Can you work these out from the model? Positions are in its coordinate system, mm. A direction names the side the tool comes from. Give positions to 0.01 mm unless a question says otherwise; leave off trailing zeros. Order: outer loops, then holes, each group sorted by start corner. A loop starts at its lowest first (then second) coordinate and runs counter-clockwise, first axis right, second up.
```python
from build123d import *

# Parameters (mm, degrees)
BOSS_EXTRUDE1_DEPTH     = 3
BOSS_EXTRUDE2_DEPTH     = 3.4
CUT_EXTRUDE1_DEPTH      = 1
CUT_EXTRUDE1_DEPTH_BACK = 8.35
CUT_EXTRUDE2_DEPTH      = 10.948718941
CUT_EXTRUDE2_DEPTH_BACK = 7
SKETCH6_R               = 1.5
SKETCH6_R_2             = 1
CUT_EXTRUDE4_DEPTH      = 1
CUT_EXTRUDE4_DEPTH_BACK = 8.35
FILLET1_R               = 10
FILLET2_R               = 3


with BuildPart() as part:
    # Sketch1 → Boss-Extrude1 (new body, symmetric)
    with BuildSketch(Plane.XY):
        Polygon((-14.712036777, 3.95), (8.397963223, 3.95), (28.677963223, 0), (-14.712036777, 0), align=None)
    extrude(amount=BOSS_EXTRUDE1_DEPTH, both=True)

    # Sketch2 → Boss-Extrude2 (add)
    with BuildSketch(Plane.XZ):
        with BuildLine():
            Line((-11.712036777, -3), (31.08325999, -3))
            Line((31.08325999, -3), (42.367258396, 7.779455791))
            ThreePointArc((42.367258396, 7.779455791), (42.464252889, 12.020987598), (38.222721082, 12.117982091))
            Line((38.222721082, 12.117982091), (28.677963223, 3))
            Line((28.677963223, 3), (-11.712036777, 3))
            ThreePointArc((-11.712036777, 3), (-14.712036777, 0), (-11.712036777, -3))
        make_face()
    extrude(amount=BOSS_EXTRUDE2_DEPTH)

    # Sketch3 → Cut-Extrude1 (cut, two sides)
    with BuildSketch(Plane(origin=(0, 3.95, 0), x_dir=(1, 0, 0), z_dir=(0, 1, 0))) as cut_extrude1_sk:
        with BuildLine():
            ThreePointArc((-14.712036777, 0), (-13.833357121, 2.121320344), (-11.712036777, 3))
            Line((-11.712036777, 3), (-14.712036777, 3))
            Line((-14.712036777, 3), (-14.712036777, 0))
        make_face()
        with BuildLine():
            ThreePointArc((-11.712036777, -3), (-13.833357121, -2.121320344), (-14.712036777, 0))
            Line((-14.712036777, 0), (-14.712036777, -3))
            Line((-14.712036777, -3), (-11.712036777, -3))
        make_face()
    extrude(amount=CUT_EXTRUDE1_DEPTH, mode=Mode.SUBTRACT)
    extrude(cut_extrude1_sk.sketch, amount=-CUT_EXTRUDE1_DEPTH_BACK, mode=Mode.SUBTRACT)

    # Sketch4 → Cut-Extrude2 (cut, two sides)
    with BuildSketch(Plane.XY.offset(3)) as cut_extrude2_sk:
        Polygon((-14.712036777, 0.25), (8.825585542, 0.25), (27.565332378, -3.4), (-14.712036777, -3.4), align=None)
    extrude(amount=CUT_EXTRUDE2_DEPTH, mode=Mode.SUBTRACT)
    extrude(cut_extrude2_sk.sketch, amount=-CUT_EXTRUDE2_DEPTH_BACK, mode=Mode.SUBTRACT)

    # Sketch6 → Cut-Extrude4 (cut, two sides)
    with BuildSketch(Plane(origin=(0, 3.95, 0), x_dir=(1, 0, 0), z_dir=(0, 1, 0))) as cut_extrude4_sk:
        with Locations((-11.712036777, 0)):
            Circle(SKETCH6_R)
        with Locations((40.294989739, -9.948718941)):
            Circle(SKETCH6_R_2)
    extrude(amount=CUT_EXTRUDE4_DEPTH, mode=Mode.SUBTRACT)
    extrude(cut_extrude4_sk.sketch, amount=-CUT_EXTRUDE4_DEPTH_BACK, mode=Mode.SUBTRACT)

    # Fillet1
    fillet1_edges = [part.edges().sort_by_distance(p)[0] for p in [
        (8.397963223, 3.95, 0),
        (28.677963223, 0, 0),
        (27.565332378, -3.4, 0),
        (8.825585542, 0.25, 0),
    ]]
    fillet(fillet1_edges, radius=FILLET1_R)

    # Fillet2
    fillet2_edges = [part.edges().sort_by_distance(p)[0] for p in [
        (31.08325999, -1.7, -3),
        (28.677963223, -1.676674581, 3),
    ]]
    fillet(fillet2_edges, radius=FILLET2_R)


solid = part.part
```
1) Suppose I cut it at B-B (x = 4.5). Please give me the cut outline in (y, z).
2) Suppose I cut it at C-C (y = 2.5). Please give me the cut outline in (x, z).
3) Suppose I cut it at A-A (y = -0.75). Please give me the cut outline in (x, z), and give its area (3 significant figures).
4) We'd pull the mould along Z, two halves only. Please class faces 4 (the face through (-4, 0.25, 0)), 5 (the face through (30.98, -1.72, -2.79)), 6 (the face through (33.946, -1.676, 8.032)), 7 (the face through (40.078, -1.676, 10.925)): +Z half, -Z half, draft (parallel to the pull), parting line (faces both ways), or undercut.
5) If I drill on line 1 (Y direction, x = -10, z = 2); line 2 (Z direction, x = 14, y = -0.5); line 3 (Y direction, x = 39, z = 12.25), over which ranges is the centre line in solid material (lowest first)?
6) Suppose I cut it at D-D (x = 19). Please give me the cut outline in (y, z) (3 decimals).
7) I'm going to push flat-ended pins straight in: pin 1 Ø1.8 at (x, z) = (-6, 0) entering from -Y; pin 2 Ø2 at (x, y) = (10.5, -1) entering from -Z; pin 3 Ø1.5 at (x, y) = (28.5, -2.5) entering from +Z; pin 4 Ø3 at (x, z) = (40.29, 9.95) entering from +Y. Where does each tip first touch, or does it pass through?
8) Which directions (+Z, -Z, +X, -X, +Y, -Y) give clear straight access to the entire face, cutting with the end or side of a thin tool? Please do faces 1 (the face through (36, 0, 5)), 2 (the face through (8, 1, 3)), 3 (the face through (37.09, -1.68, 2.74)).
Results:
1. outline: (0.25, -3) - (3.95, -3) - (3.95, 3) - (0.25, 3) - close
2. outline: (-11.71, -3) - (15.84, -3) - (15.84, 3) - (-11.71, 3) arc R3 ccw to start; hole circle Ø3 at (-11.71, 0)
3. outline: (13.96, -3) - (29.88, -3) arc R3 ccw to (31.95, -2.17) - (42.37, 7.78) arc R3 ccw to (38.22, 12.12) - (29.55, 3.83) arc R3 cw to (27.48, 3) - (13.96, 3) - close; hole circle Ø2 at (40.29, 9.95)
3. area: 193 mm2
4. face 4: draft
4. face 5: -Z half
4. face 6: +Z half
4. face 7: undercut
5. line 1: y = 0.25 to 3.95
5. line 2: z = -3 to 3
5. line 3: y = -3.4 to 0
6. outline: (-1.732, -3) - (1.885, -3) - (1.885, 3) - (-1.732, 3) - close
7. pin 1: stops at y = 0.25
7. pin 2: stops at z = -3
7. pin 3: stops at z = 3.58
7. pin 4: stops at y = 0
8. face 1: +Z, -Z, +X, +Y
8. face 2: +Z, -X, +Y, -Y
8. face 3: -Z, +X, +Y, -Y
